Geometry: see drawing. Coordinates: mm, zero at the bounding-box minimum. Round coordinates to 2 decimals unless told otherwise and drop trailing zeros. Loops run counter-clockwise (first coordinate to the right, second up) from the corner with the lowest first, then second, coordinate; pieces in that order, holes last.
(1) Section A-A, the plane x = 90.5. Return the cut outline in (y, z), plus the area to 3 significant figures.
(2) Material intervals for probe 1 along X at (y, z) = (20.5, 0.7); probe 2 along X at (y, z) = (39.5, 2.85); probe 3 along Y at (x, z) = (55, 0.5), sorted ascending.
(3) Section C-C, the plane z = 1.4. Return the cut outline in (x, y), plus the area to 3 significant figures.
(4) First-contact query: pin 1 Ø1.5 at (y, z) = (24, 2) entering from -X; pin 2 Ø1.5 at (x, z) = (47, 2) entering from -Y; pin 3 Ø0.9 at (y, z) = (32, 1.5) entering from +X. Flat tips, straight axial feed; report the tip coordinate or a pass-through.
(5) Section D-D, the plane x = 179. Return the cut outline in (y, z), plus the area to 3 significant figures.
(6) Section B-B, the plane y = 41. Return the cut outline in (x, z), plus the area to 3 significant figures.
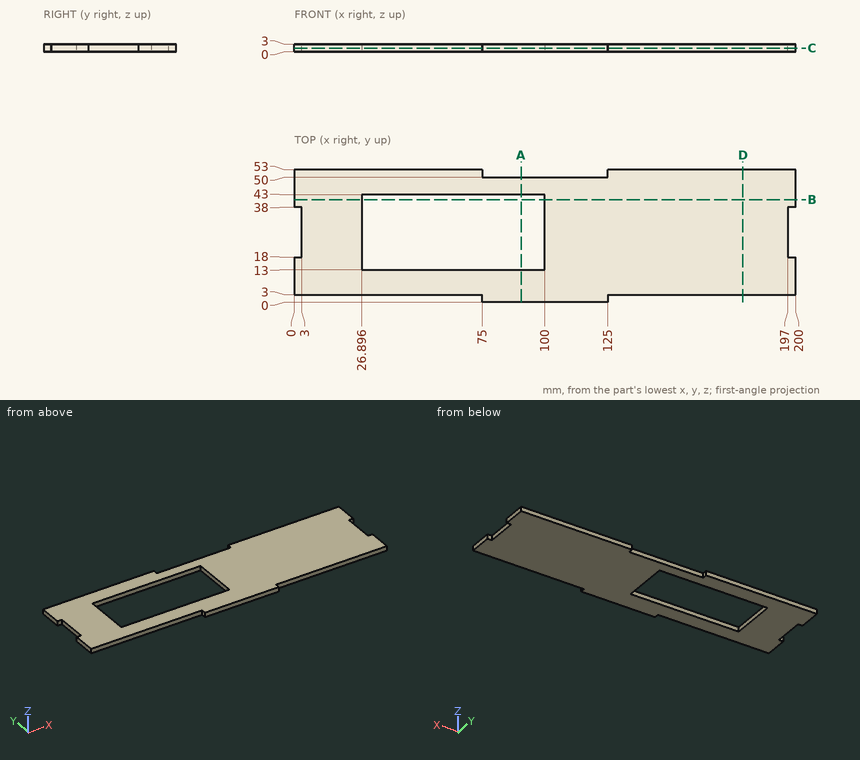
Output values:
1. outline: (0, 0) - (13, 0) - (13, 3) - (0, 3) - close; (43, 0) - (50, 0) - (50, 3) - (43, 3) - close
1. area: 60.0 mm2
2. probe 1: x = 3 to 26.9, 100 to 197
2. probe 2: x = 0 to 26.9, 100 to 200
2. probe 3: y = 3 to 13, 43 to 53
3. outline: (0, 3) - (75, 3) - (75, 0) - (125, 0) - (125, 3) - (200, 3) - (200, 18) - (197, 18) - (197, 38) - (200, 38) - (200, 53) - (125, 53) - (125, 50) - (75, 50) - (75, 53) - (0, 53) - (0, 38) - (3, 38) - (3, 18) - (0, 18) - close; hole (26.9, 13) - (100, 13) - (100, 43) - (26.9, 43) - close
3. area: 7,690 mm2
4. pin 1: stops at x = 3
4. pin 2: stops at y = 3
4. pin 3: stops at x = 197
5. outline: (3, 0) - (53, 0) - (53, 3) - (3, 3) - close
5. area: 150 mm2
6. outline: (0, 0) - (26.9, 0) - (26.9, 3) - (0, 3) - close; (100, 0) - (200, 0) - (200, 3) - (100, 3) - close
6. area: 381 mm2
